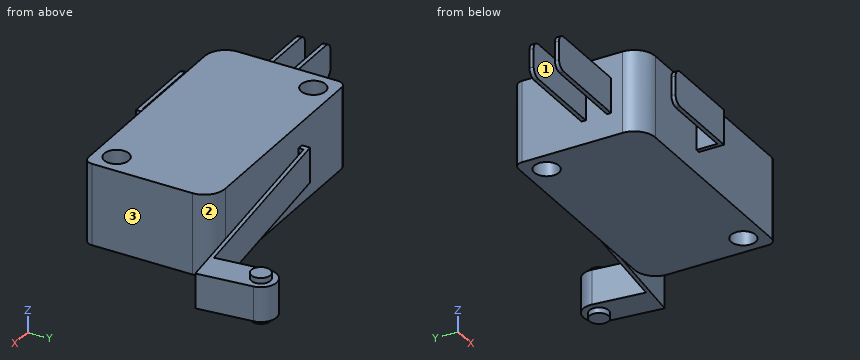
from build123d import *

# Parameters (mm, degrees)
SKETCH1_W                = 27.94
SKETCH1_H                = 15.748
BOSS_EXTRUDE1_DEPTH      = 9.906
SKETCH2_R                = 1.49225
CUT_EXTRUDE1_DEPTH       = 34.567423792
FILLET1_R                = 2.54
BOSS_EXTRUDE2_DEPTH      = 2.1209
BOSS_EXTRUDE2_DEPTH_BACK = 2.1209
SKETCH3_W                = 10.922
SKETCH3_H                = 0.508
FILLET2_R                = 1
BOSS_EXTRUDE3_DEPTH      = 2.794
BOSS_EXTRUDE3_DEPTH_BACK = 2.794
SKETCH4_R                = 1.155


with BuildPart() as part:
    # Sketch1 → Boss-Extrude1 (new body)
    with BuildSketch(Plane.XY):
        with Locations((13.97, 7.874)):
            Rectangle(SKETCH1_W, SKETCH1_H)
    extrude(amount=BOSS_EXTRUDE1_DEPTH)

    # Sketch2 → Cut-Extrude1 (cut, through all)
    with BuildSketch(Plane.XY.offset(9.906)):
        with Locations((2.54, 13.208)):
            Circle(SKETCH2_R)
        with Locations((25.4, 2.54)):
            Circle(SKETCH2_R)
    extrude(amount=-CUT_EXTRUDE1_DEPTH, mode=Mode.SUBTRACT)

    # Fillet1
    fillet1_edges = [part.edges().sort_by_distance(p)[0] for p in [
        (27.94, 15.748, 4.953),
        (0, 0, 4.953),
    ]]
    fillet(fillet1_edges, radius=FILLET1_R)

    # Sketch3 → Boss-Extrude2 (add, two sides: drawn at the far end of the back side and taken through both)
    with BuildSketch(Plane.XY.offset(4.953).offset(-BOSS_EXTRUDE2_DEPTH_BACK)):
        with BuildLine():
            Line((9.321868026, 15.748), (9.321868026, 16.736327505))
            Line((9.321868026, 16.736327505), (34.261319398, 19.503534314))
            Line((34.261319398, 19.503534314), (33.574009344, 25.69791617))
            ThreePointArc((33.574009344, 25.69791617), (35.257306032, 27.801380518), (37.360770379, 26.11808383))
            Line((37.360770379, 26.11808383), (38.1, 19.455776874))
            Line((38.1, 19.455776874), (10.0081978, 16.338794661))
            Line((10.0081978, 16.338794661), (10.0081978, 15.748))
            Line((10.0081978, 15.748), (9.321868026, 15.748))
        make_face()
        Polygon((11.178880787, 0), (11.178880787, -2.54), (1.526880787, -2.54), (1.526880787, -3.048), (11.686880787, -3.048), (11.686880787, 0), align=None)
        with Locations((-5.461, 4.149928027)):
            Rectangle(SKETCH3_W, SKETCH3_H)
        with Locations((-5.461, 7.23359273)):
            Rectangle(SKETCH3_W, SKETCH3_H)
    extrude(amount=BOSS_EXTRUDE2_DEPTH + BOSS_EXTRUDE2_DEPTH_BACK)

    # Fillet2
    fillet2_edges = [part.edges().sort_by_distance(p)[0] for p in [
        (1.526880787, -2.794, 2.8321),
        (1.526880787, -2.794, 7.0739),
        (-10.922, 4.149928027, 2.8321),
        (-10.922, 4.149928027, 7.0739),
        (0, 15.748, 4.953),
        (27.94, 0, 4.953),
        (-10.922, 7.23359273, 2.8321),
        (-10.922, 7.23359273, 7.0739),
    ]]
    fillet(fillet2_edges, radius=FILLET2_R)

    # Sketch4 → Boss-Extrude3 (add, two sides: drawn at the far end of the back side and taken through both)
    with BuildSketch(Plane.XY.offset(4.953).offset(-BOSS_EXTRUDE3_DEPTH_BACK)):
        with Locations((35.467389862, 25.908)):
            Circle(SKETCH4_R)
    extrude(amount=BOSS_EXTRUDE3_DEPTH + BOSS_EXTRUDE3_DEPTH_BACK)


solid = part.part
The listing builds one solid part. Answer for the finished solid, in the listing's coordinates (mm). Face numbers are marked on the shaded views. A direction names the side the tool comes from. Coordinates: 2 decimals unless noted, no trailing zeros. Order: outer loops, then holes, each group sorted by start corner. A loop starts at its lowest first (then second) coordinate and runs counter-clockwise, first axis right, second up.
Q1. Which of the six approach directions +Z, -Z, +X, -X, +Y, -Y give full straight-line access (tool end or side, diameter ignored) to the marked faces 1, 2 and 3?
Q2. A cutting plane is placed at A-A, the plane z = 8.75. Write down the section's boundary in (x, y).
Q3. A cutting plane is placed at B-B, the plane y = -1. Write down the section's boundary in (x, z).
Q4. A cutting plane is placed at C-C, the plane x = 33. Write down the section's boundary in (y, z).
Q5. Consider line 1 (Y direction, x = 2.54, z = 3.5); line 2 (Y direction, x = -5, z = 4.75); line 3 (X direction, y = 9, z = 0.5). Determine where each line is inside the solid, lowest interval first.
Q6. Given P1, Ø1, axis at x = -2, z = 5, coming from the +Y side; P2, Ø1, axis at y = 21.5, z = 5, coming from the +X side; P3, Ø5, axis at x = 13.5, z = 4.5, coming from the +Y side; P4, Ø0.9, axis at x = 7.5, y = -1, coming from the -Z side, each flat-ended and moving along its own axis, determine where each tip first touches the part or whether it passes through.
Answers follow:
1. face 1: +Z, -Z, -X
1. face 2: +Z, -Z, +X
1. face 3: +Z, -Z, +X, -Y
2. outline: (0, 2.54) arc R2.54 ccw to (2.54, 0) - (26.94, 0) arc R1 ccw to (27.94, 1) - (27.94, 13.21) arc R2.54 ccw to (25.4, 15.75) - (1, 15.75) arc R1 ccw to (0, 14.75) - close; hole circle Ø2.98 at (2.54, 13.21); hole circle Ø2.98 at (25.4, 2.54)
3. outline: (11.18, 2.83) - (11.69, 2.83) - (11.69, 7.07) - (11.18, 7.07) - close
4. outline: (18.89, 2.83) - (19.36, 2.83) - (19.36, 7.07) - (18.89, 7.07) - close
5. line 1: y = -3.05 to -2.54, 0 to 11.72, 14.7 to 15.75
5. line 2: y = 3.9 to 4.4, 6.98 to 7.49
5. line 3: x = 0 to 27.94
6. P1: stops at y = 7.49
6. P2: stops at x = 37.93
6. P3: stops at y = 17.48
6. P4: passes through
